Geometry check sheet. Reference: the model listing, model coordinates, mm. Give positions to 0.01 mm unless a question says otherwise; leave off trailing zeros. Order: outer loops, then holes, each group sorted by start corner. A loop starts at its lowest first (then second) coordinate and runs counter-clockwise, first axis right, second up. Notation, with made-up numbers: M 78.25,80 L 89.25,80 A16 ccw 89.25,106 Z; hole C 59.5,-10.75 d7. An arc over 180 degrees is marked long. Use CSV: the item, a comma, the result in double quotes. Start each with the question number.
from build123d import *

# Parameters (mm, degrees)
SKETCH1_R           = 1.5
BOSS_EXTRUDE1_DEPTH = 20.5
SKETCH2_R           = 2
BOSS_EXTRUDE2_DEPTH = 1
SKETCH3_R           = 2
BOSS_EXTRUDE3_DEPTH = 1
FILLET1_R           = 0.5


with BuildPart() as part:
    # Sketch1 → Boss-Extrude1 (new body)
    with BuildSketch(Plane.XY):
        Circle(SKETCH1_R)
    extrude(amount=BOSS_EXTRUDE1_DEPTH)

    # Sketch2 → Boss-Extrude2 (add)
    with BuildSketch(Plane(origin=(0, 0, 0), x_dir=(-1, 0, 0), z_dir=(0, 0, -1))):
        Circle(SKETCH2_R)
    extrude(amount=BOSS_EXTRUDE2_DEPTH)

    # Sketch3 → Boss-Extrude3 (add)
    with BuildSketch(Plane.XY.offset(20.5)):
        Circle(SKETCH3_R)
    extrude(amount=BOSS_EXTRUDE3_DEPTH)

    # Fillet1
    fillet1_edges = [part.edges().sort_by_distance(p)[0] for p in [
        (-2, 0, 21.5),
        (2, 0, -1),
    ]]
    fillet(fillet1_edges, radius=FILLET1_R)


solid = part.part
(1) Thickness scan on line 1 (Z direction, x = 0.7, y = -1.4); line 2 (Z direction, x = 0.65, y = 1.65); line 3 (X direction, y = -0.1, z = 14). Record the ranges inside material, lowest first.
(2) Go/stop test with flat-tipped pins: P1, Ø2, axis at y = -1.5, z = 18.5, coming from the +X side; P2, Ø1, axis at x = 0.5, z = 2, coming from the -Y side; P3, Ø2, axis at y = 1, z = 6.5, coming from the +X side. Record where each tip stops, or that it passes through.
(3) Sectioned sample at A-A on x = 0. Record the cut outline in (y, z).
(4) Sectioned sample at C-C on z = 15.75. Record the cut outline in (x, y).
(5) Draft check along Z on faces 1 (the face through (0, 0, 21.5)), 2 (the face through (-1.5, 0.07, 10.11)), 3 (the face through (0, 0, -1)), 4 (the face through (-0.434, -1.952, 20.746)). Enter one of: +Z half, -Z half, draft (parallel to the pull), parting line (faces both ways), or undercut.
Responses:
1,line 1,"-1 to 0, 20.5 to 21.5"
1,line 2,"-0.92 to 0, 20.5 to 21.42"
1,line 3,"-1.5 to 1.5"
2,P1,"x = 1.41"
2,P2,"y = -1.5"
2,P3,"x = 1.5"
3,outline,"M -2,-0.5 A0.5 ccw -1.5,-1 L 1.5,-1 A0.5 ccw 2,-0.5 L 2,0 L 1.5,0 L 1.5,20.5 L 2,20.5 L 2,21 A0.5 ccw 1.5,21.5 L -1.5,21.5 A0.5 ccw -2,21 L -2,20.5 L -1.5,20.5 L -1.5,0 L -2,0 Z"
4,outline,"C 0,0 d3"
5,face 1,"+Z half"
5,face 2,"undercut"
5,face 3,"-Z half"
5,face 4,"draft"
